Study the drawing (mm; zero at the part's minimum x, y, z) and answer. A direction names the side the tool comes from. Give positions to 0.01 mm unless a question says otherwise; leave off trailing zeros. Loops run counter-clockwise (first coordinate to the right, second up) from the corner with the lowest first, then second, coordinate; pieces in that order, holes last. Notation, with made-up numbers: (44, 53.5) - (79, 53.5) arc R15 cw to (79, 79.5) - close; hole circle Ø7 at (47, -14.75). An arc over 180 degrees is marked (long way). Use one line per item in the form item = value. Start each with the question number.
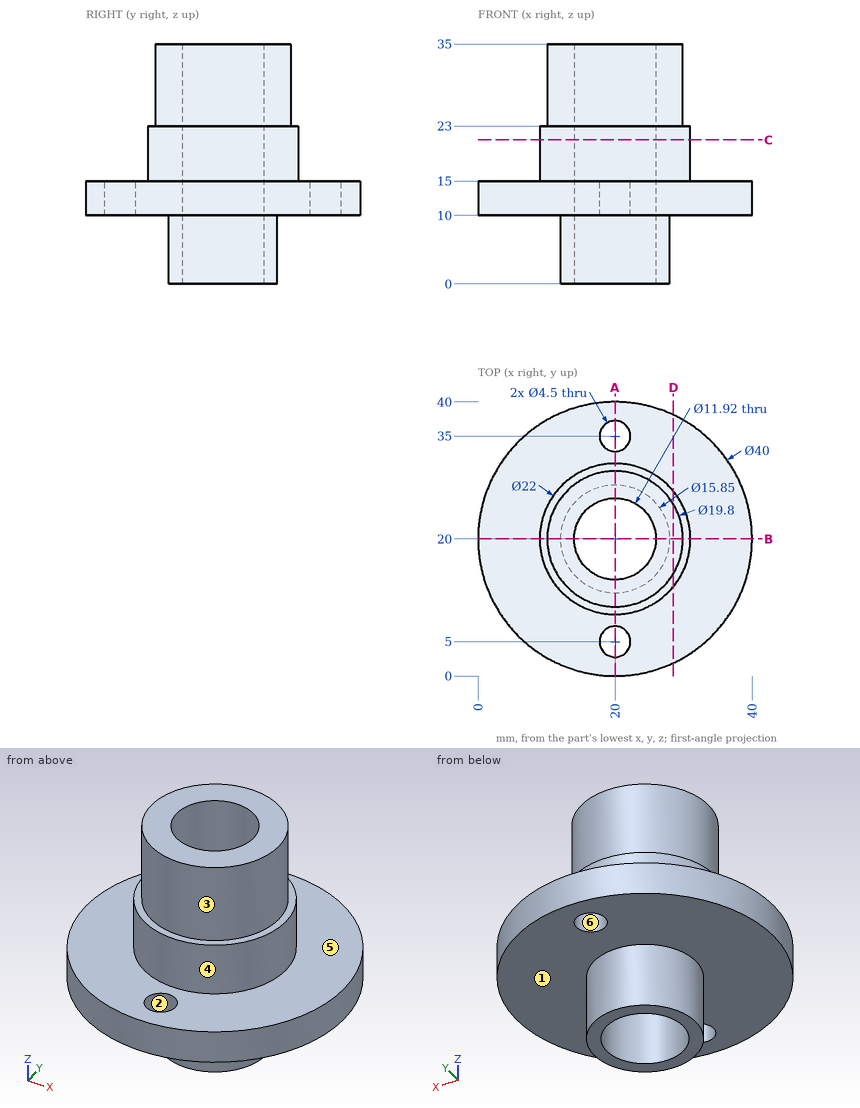
1) A tool of negligible diameter and unlimited length cuts with its end or side. For the marked faces 1, 2 and 3, from which of +Z, -Z, +X, -X, +Y, -Y can it reach the whole face along a straight path? Write none if from no direction.
2) A cutting plane is placed at B-B (y = 20). Give the vertices of the cut face in (x, z) (3 decimals), plus the area to 3 significant figures.
3) A cutting plane is placed at A-A (x = 20). Give the vertices of the cut face in (y, z) (3 decimals), plus the area to 3 significant figures.
4) A cutting plane is placed at D-D (x = 28.5). Give the vertices of the cut face in (y, z).
5) A cutting plane is placed at C-C (z = 21). Give the vertices of the cut face in (x, y).
6) Determine the mould class of the marked faces 4, 5 and 6 for opening direction X: released by +X, released by -X, zero draft, split by the parting line, or undercut.
7) Flat-ended cylindrical pins translate along their axes: pin 1 Ø5 at (x, z) = (33.5, 7) entering from +Y; pin 2 Ø5 at (x, y) = (20, 5) entering from -Z; pin 3 Ø2 at (y, z) = (16.5, 23.5) entering from -X; pin 4 Ø1 at (x, z) = (13, 29.5) entering from +Y. Find the tip coordinate at first contact, or state that the pin passes through.
8) Find the intervals of material crossed by probe 1 along Y at (x, z) = (20, 12); probe 2 along Y at (x, z) = (20, 26); probe 3 along Z at (x, y) = (12, 26), in increasing order.
Answer sheet:
q1.face_1 = -Z
q1.face_2 = +Z, -Z
q1.face_3 = +Z
q2.outline = (0, 10) - (12.075, 10) - (12.075, 0) - (14.04, 0) - (14.04, 35) - (10.1, 35) - (10.1, 23) - (9, 23) - (9, 15) - (0, 15) - close; (25.96, 0) - (27.925, 0) - (27.925, 10) - (40, 10) - (40, 15) - (31, 15) - (31, 23) - (29.9, 23) - (29.9, 35) - (25.96, 35) - close
q2.area = 355 mm²
q3.outline = (0, 10) - (2.75, 10) - (2.75, 15) - (0, 15) - close; (7.25, 10) - (12.075, 10) - (12.075, 0) - (14.04, 0) - (14.04, 35) - (10.1, 35) - (10.1, 23) - (9, 23) - (9, 15) - (7.25, 15) - close; (25.96, 0) - (27.925, 0) - (27.925, 10) - (32.75, 10) - (32.75, 15) - (31, 15) - (31, 23) - (29.9, 23) - (29.9, 35) - (25.96, 35) - close; (37.25, 10) - (40, 10) - (40, 15) - (37.25, 15) - close
q3.area = 310 mm²
q4.outline = (1.9, 10) - (38.1, 10) - (38.1, 15) - (26.98, 15) - (26.98, 23) - (25.08, 23) - (25.08, 35) - (14.92, 35) - (14.92, 23) - (13.02, 23) - (13.02, 15) - (1.9, 15) - close
q5.outline = circle Ø22 at (20, 20); hole circle Ø11.92 at (20, 20)
q6.face_4 = split by the parting line
q6.face_5 = zero draft
q6.face_6 = undercut
q7.pin_1 = through
q7.pin_2 = 10
q7.pin_3 = 9.32
q7.pin_4 = 27.47
q8.probe_1 = 0 to 2.75, 7.25 to 14.04, 25.96 to 32.75, 37.25 to 40
q8.probe_2 = 10.1 to 14.04, 25.96 to 29.9
q8.probe_3 = 10 to 23
